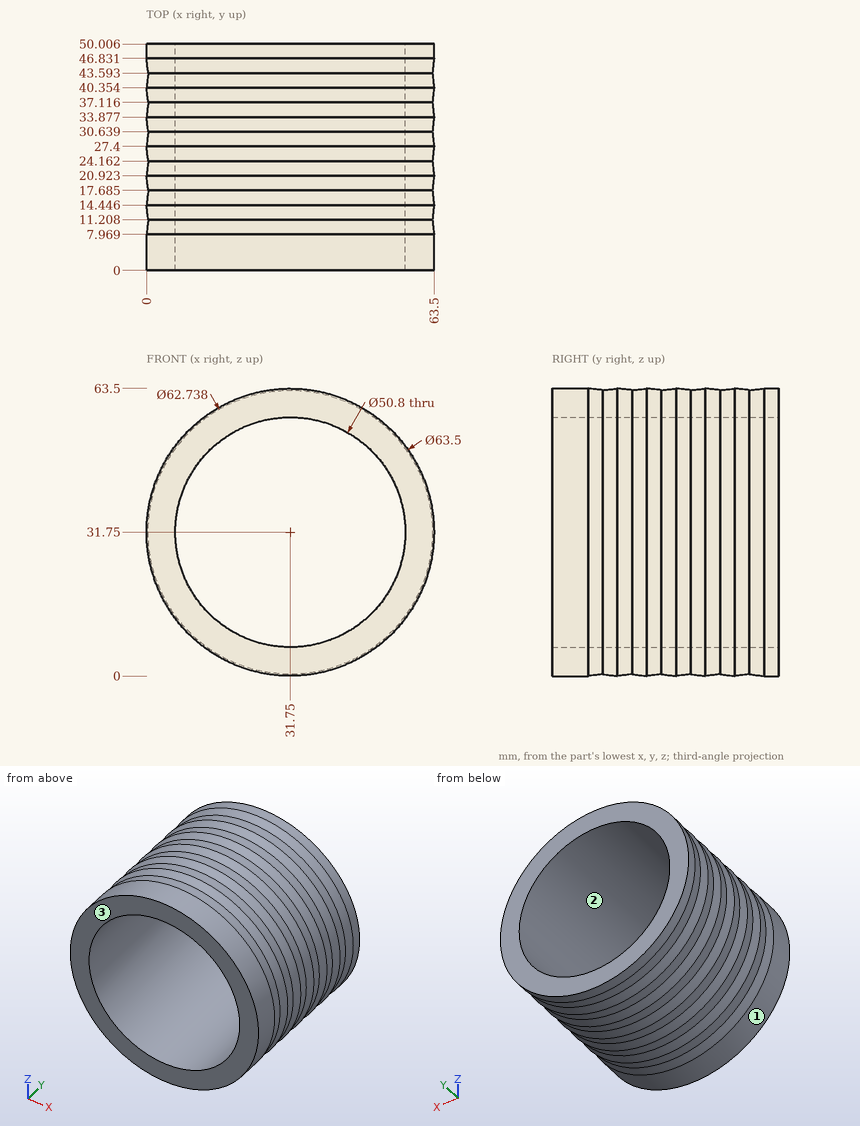
Verification items for this drawing (mm, ordinates from the low corner). Coordinates: 2 decimals unless noted, no trailing zeros. Use CSV: the item, a comma, the result in double quotes. Start each with the question number.
Item 1: Mould release check, pull along X, two halves, no side actions. Record for the marked faces 1, 2 and 3: released by +X, released by -X, zero draft, split by the parting line, or undercut.
Item 2: Depth check by flat-ended pin: pin 1 Ø4 at (x, y) = (24.5, 21.5) entering from +Z; pin 2 Ø1.5 at (x, y) = (40.5, 28) entering from +Z; pin 3 Ø4 at (x, y) = (27, 26) entering from -Z. Enter the tip coordinate at first touch or a pass-through.
Item 3: Thickness scan on line 1 (Z direction, x = 31, y = 34); line 2 (X direction, y = 37.5, z = 31.75); line 3 (X direction, y = 19.5, z = 54) (1 decimal). Record the ranges inside material, lowest first.
Answers:
1,face 1,"split by the parting line"
1,face 2,"undercut"
1,face 3,"zero draft"
2,pin 1,"z = 63.05"
2,pin 2,"z = 62.42"
2,pin 3,"z = 0.17"
3,line 1,"0.02 to 6.36, 57.14 to 63.48"
3,line 2,"0.34 to 6.35, 57.15 to 63.16"
3,line 3,"9.3 to 19.5, 44 to 54.2"
